Source: CAD feature listing. Evaluate the final solid. Frame: model axes, mm. A direction names the side the tool comes from. Give positions to 0.01 mm unless a question says otherwise; leave off trailing zeros. Loops run counter-clockwise (first coordinate to the right, second up) from the corner with the lowest first, then second, coordinate; pieces in that order, holes last.
```python
from build123d import *

# Parameters (mm, degrees)
F0_W      = 78
F0_H      = 78
F1_DEPTH  = 8
F2_R      = 7
F3_R      = 4
F4_DEPTH  = 8.001
F5_R      = 35
F6_DEPTH  = 22
F7_R      = 33
F8_DEPTH  = 4
F10_R     = 0.6
F13_DEPTH = 21
F14_R     = 7.5
F15_DEPTH = 25
F16_R     = 11
F17_DEPTH = 14
F18_R     = 11
F19_DEPTH = 9
F20_R     = 7
F21_DEPTH = 35.001
F22_R     = 7
F23_DEPTH = 40.001


with BuildPart() as f1:
    # F0 (on Front) → F1 (new body)
    with BuildSketch(Plane.XZ):
        with Locations((0, 39)):
            Rectangle(F0_W, F0_H)
    extrude(amount=F1_DEPTH)

    # F2
    f2_edges = [f1.edges().sort_by_distance(p)[0] for p in [
        (-39, -4, 78),
        (39, -4, 78),
        (39, -4, 0),
        (-39, -4, 0),
    ]]
    fillet(f2_edges, radius=F2_R)

    # F3 (on face) → F4 (cut, through all)
    with BuildSketch(Plane.XZ.offset(8)):
        with Locations((-32, 71)):
            Circle(F3_R)
        with Locations((32, 71)):
            Circle(F3_R)
        with Locations((-32, 7)):
            Circle(F3_R)
        with Locations((32, 7)):
            Circle(F3_R)
    extrude(amount=-F4_DEPTH, mode=Mode.SUBTRACT)

    # F5 (on face) → F6 (join)
    with BuildSketch(Plane.XZ.offset(8)):
        with Locations((0, 39)):
            Circle(F5_R)
    extrude(amount=F6_DEPTH)

    # F7 (on face) → F8 (cut)
    with BuildSketch(Plane.XZ.offset(30)):
        with Locations((0, 39)):
            Circle(F7_R)
    extrude(amount=-F8_DEPTH, mode=Mode.SUBTRACT)

    # F11: sweep along a path in F9
    with BuildLine(Plane(origin=(0, 0, 0), x_dir=(-1, 0, 0), z_dir=(0, 1, 0))) as f11_path:
        CenterArc((0, 39), 35, 0, 360)
    # F10 (on Right) → F11 (sweep, cut)
    with BuildSketch(Plane.YZ):
        with Locations((0, 74)):
            Circle(F10_R)
    sweep(path=f11_path.line, mode=Mode.SUBTRACT)

    # F12 (on face) → F13 (cut)
    with BuildSketch(Plane(origin=(0, 0, 0), x_dir=(-1, 0, 0), z_dir=(0, 1, 0))):
        with BuildLine():
            ThreePointArc((0, 28.8387992835), (18.3735463151, 23.3995192382), (29.5, 39))
            ThreePointArc((29.5, 39), (18.3735463151, 54.6004807618), (0, 49.1612007165))
            ThreePointArc((0, 49.1612007165), (2.6004807618, 44.3735463151), (3.5, 39))
            ThreePointArc((3.5, 39), (2.6004807618, 33.6264536849), (0, 28.8387992835))
        make_face()
        with BuildLine():
            ThreePointArc((3.5, 39), (2.6004807618, 44.3735463151), (0, 49.1612007165))
            ThreePointArc((0, 49.1612007165), (-3.5, 39), (0, 28.8387992835))
            ThreePointArc((0, 28.8387992835), (2.6004807618, 33.6264536849), (3.5, 39))
        make_face()
        with BuildLine():
            ThreePointArc((0, 28.8387992835), (-3.5, 39), (0, 49.1612007165))
            ThreePointArc((0, 49.1612007165), (-29.5, 39), (0, 28.8387992835))
        make_face()
    extrude(amount=-F13_DEPTH, mode=Mode.SUBTRACT)

    # F14 (on face) → F15 (cut)
    with BuildSketch(Plane(origin=(0, 0, 0), x_dir=(-1, 0, 0), z_dir=(0, 1, 0))):
        with Locations((0, 28.3387992835)):
            Circle(F14_R)
        with Locations((0, 49.6612007165)):
            Circle(F14_R)
    extrude(amount=-F15_DEPTH, mode=Mode.SUBTRACT)

    # F16 (on face) → F17 (join)
    with BuildSketch(Plane.XZ.offset(26)):
        with Locations((13, 39)):
            Circle(F16_R)
    extrude(amount=F17_DEPTH)

    # F18 (on face) → F19 (join)
    with BuildSketch(Plane.XZ.offset(26)):
        with Locations((-13, 39)):
            Circle(F18_R)
    extrude(amount=F19_DEPTH)

    # F20 (on face) → F21 (cut, through all)
    with BuildSketch(Plane.XZ.offset(35)):
        with Locations((-13, 39)):
            Circle(F20_R)
    extrude(amount=-F21_DEPTH, mode=Mode.SUBTRACT)

    # F22 (on face) → F23 (cut, through all)
    with BuildSketch(Plane.XZ.offset(40)):
        with Locations((13, 39)):
            Circle(F22_R)
    extrude(amount=-F23_DEPTH, mode=Mode.SUBTRACT)


solid = f1.part
```
(1) Section D-D, the plane y = -17. Return the cut outline in (x, z).
A:
outline: circle Ø70 at (0, 39); hole (-6.12, 24) arc R7.5 ccw to (6.12, 24) arc R16.5 ccw (long way) to (6.12, 54) arc R7.5 ccw to (-6.12, 54) arc R16.5 ccw (long way) to start
(2) Section A-A, the plane x = 0. Return the cut outline in (y, z).
A:
outline: (-30, 4) - (-8, 4) - (-8, 0) - (0, 0) - (0, 3.4) arc R0.6 cw to (0, 4.6) - (0, 20.84) - (-25, 20.84) - (-25, 35.84) - (-21, 35.84) - (-21, 42.16) - (-25, 42.16) - (-25, 57.16) - (0, 57.16) - (0, 73.4) arc R0.6 cw to (0, 74.6) - (0, 78) - (-8, 78) - (-8, 74) - (-30, 74) - (-30, 72) - (-26, 72) - (-26, 6) - (-30, 6) - close
(3) Section B-B, the plane y = -5.5. Return the cut outline in (x, z), then the cut area to 3 significant figures.
A:
outline: (-39, 7) arc R7 ccw to (-32, 0) - (32, 0) arc R7 ccw to (39, 7) - (39, 71) arc R7 ccw to (32, 78) - (-32, 78) arc R7 ccw to (-39, 71) - close; hole circle Ø8 at (-32, 7); hole circle Ø8 at (-32, 71); hole (-6.12, 24) arc R7.5 ccw to (6.12, 24) arc R16.5 ccw (long way) to (6.12, 54) arc R7.5 ccw to (-6.12, 54) arc R16.5 ccw (long way) to start; hole circle Ø8 at (32, 7); hole circle Ø8 at (32, 71)
area: 4,120 mm2
(4) First-contact query: pin 1 (13.5 mm diameter, centred on x = 0, z = 49.66, fed in from +Y); pin 2 (13 mm diameter, centred on x = -32, z = 7, fed in from -Y); pin 3 (1.5 mm diameter, centred on y = -13, z = 27.5, fed in from -X). Flat tips, straight axial feed; report the tip coordinate or a pass-through.
A:
pin 1: stops at y = -25
pin 2: stops at y = -8
pin 3: stops at x = -33.31
(5) Ray query, line 1 along Z through (x, y) = (32, -1.5); line 2 along Z through (x, y) = (0, -28); line 3 along Z through (x, y) = (-13, -31). Return the intervals inside material, ascending.
A:
line 1: z = 0 to 3, 11 to 67, 75 to 78
line 2: z = 4 to 6, 72 to 74
line 3: z = 28 to 32, 46 to 50
(6) Mould query, pull axis Z, two halves, no side actions, for faces 1 (the flat face through (-5.8, -35, 39.2)), 2 (the cylindrical face through (37, -4.1, 75.9)), 3 (the cylindrical face through (36.9, -4.1, 2)), 4 (the cylindrical face through (-14.432, -30.437, 49.906)). Classes: pulls with the +Z half, pulls with the -Z half, needs draft (parallel to the pull), parting line crosses it, or undercut.
A:
face 1: needs draft
face 2: pulls with the +Z half
face 3: pulls with the -Z half
face 4: undercut
(7) Reachability of faces 5 (the cylindrical face through (-4.56, -18.85, 73.7)), 6 (the cylindrical face through (-37, -4.1, 2.1)), 7 (the cylindrical face through (29.494, -10.353, 39.462)) from +Z, -Z, +X, -X, +Y, -Y: full face, straight path, thin tool, end or side. Return the list, or none.
A:
face 5: -Y
face 6: -Z, -X, +Y, -Y
face 7: +Y
(8) Section C-C, the plane z = 68.5. Count the separate pieces of the cut face and the enclosed holes in it, then the cut area to 3 significant figures.
A:
separate pieces: 3
enclosed holes: 0
area: 1,230 mm2
